```python
from build123d import *

# Parameters (mm, degrees)
EXTRUDE_THIN1_OUTLINE_W   = 1485.9
EXTRUDE_THIN1_OUTLINE_H   = 1041.4
EXTRUDE_THIN1_OUTLINE_W_2 = 228.6
EXTRUDE_THIN1_OUTLINE_H_2 = 228.6
EXTRUDE_THIN1_OUTLINE_W_3 = 355.6
EXTRUDE_THIN1_OUTLINE_H_3 = 482.6
EXTRUDE_THIN1_DEPTH       = 304.8
SKETCH1_5_W               = 1460.5
SKETCH1_5_H               = 1016
BOSS_EXTRUDE1_DEPTH       = 2.54
CUT_EXTRUDE1_DEPTH        = 25.4
SKETCH4_W                 = 127
SKETCH4_H                 = 228.6
CUT_EXTRUDE2_DEPTH        = 25.4
SKETCH5_W                 = 127
SKETCH5_H                 = 228.6
CUT_EXTRUDE3_DEPTH        = 25.4
SKETCH6_W                 = 127
SKETCH6_H                 = 228.6
CUT_EXTRUDE4_DEPTH        = 25.4


# Read off the part's stored shape, not the designer's step: Extrude-Thin1
with BuildPart() as part:
    # Extrude-Thin1 outline → Extrude-Thin1 (new body)
    with BuildSketch(Plane(origin=(0, 0, 0), x_dir=(1, 0, 0), z_dir=(0, 1, 0))):
        Rectangle(EXTRUDE_THIN1_OUTLINE_W, EXTRUDE_THIN1_OUTLINE_H)
        with Locations((222.25, -381)):
            Rectangle(EXTRUDE_THIN1_OUTLINE_W_2, EXTRUDE_THIN1_OUTLINE_H_2, mode=Mode.SUBTRACT)
        with Locations((539.75, -254)):
            Rectangle(EXTRUDE_THIN1_OUTLINE_W_3, EXTRUDE_THIN1_OUTLINE_H_3, mode=Mode.SUBTRACT)
        Polygon((-44.45, 495.3), (-44.45, 241.3), (336.55, 241.3), (336.55, -241.3), (82.55, -241.3), (82.55, -495.3), (-717.55, -495.3), (-717.55, 495.3), align=None, mode=Mode.SUBTRACT)
        with Locations((539.75, 254)):
            Rectangle(EXTRUDE_THIN1_OUTLINE_W_3, EXTRUDE_THIN1_OUTLINE_H_3, mode=Mode.SUBTRACT)
        with Locations((158.75, 381)):
            Rectangle(EXTRUDE_THIN1_OUTLINE_W_3, EXTRUDE_THIN1_OUTLINE_H_2, mode=Mode.SUBTRACT)
    extrude(amount=EXTRUDE_THIN1_DEPTH)

    # Sketch1<5> → Boss-Extrude1 (add)
    with BuildSketch(Plane(origin=(0, 0, 0), x_dir=(1, 0, 0), z_dir=(0, 1, 0))):
        Rectangle(SKETCH1_5_W, SKETCH1_5_H)
    extrude(amount=BOSS_EXTRUDE1_DEPTH)

    # Sketch2 → Cut-Extrude1 (cut)
    with BuildSketch(Plane.ZY.offset(742.95)):
        Polygon((-63.5, 0), (-63.5, 228.6), (63.5, 228.6), (63.5, 0), (0, 0), align=None)
    extrude(amount=-CUT_EXTRUDE1_DEPTH, mode=Mode.SUBTRACT)

    # Sketch4 → Cut-Extrude2 (cut)
    with BuildSketch(Plane.ZY.offset(-336.55)):
        with Locations((-127, 116.84)):
            Rectangle(SKETCH4_W, SKETCH4_H)
        with Locations((127, 116.84)):
            Rectangle(SKETCH4_W, SKETCH4_H)
    extrude(amount=-CUT_EXTRUDE2_DEPTH, mode=Mode.SUBTRACT)

    # Sketch5 → Cut-Extrude3 (cut)
    with BuildSketch(Plane(origin=(0, 0, 241.3), x_dir=(-1, 0, 0), z_dir=(0, 0, -1))):
        with Locations((-209.55, 116.84)):
            Rectangle(SKETCH5_W, SKETCH5_H)
    extrude(amount=-CUT_EXTRUDE3_DEPTH, mode=Mode.SUBTRACT)

    # Sketch6 → Cut-Extrude4 (cut)
    with BuildSketch(Plane.XY.offset(-241.3)):
        with Locations((82.55, 116.84)):
            Rectangle(SKETCH6_W, SKETCH6_H)
    extrude(amount=-CUT_EXTRUDE4_DEPTH, mode=Mode.SUBTRACT)


solid = part.part
```
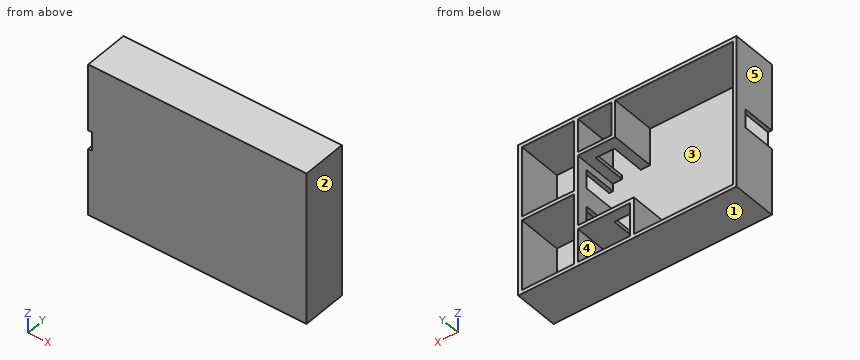
Build history of the part. All positions in model axes, mm. Face numbers are marked on the shaded views. A direction names the side the tool comes from. Round coordinates to 2 decimals unless told otherwise and drop trailing zeros. Order: outer loops, then holes, each group sorted by start corner. A loop starts at its lowest first (then second) coordinate and runs counter-clockwise, first axis right, second up. Notation, with made-up numbers: (85.25, 63.5) - (102.25, 63.5) arc R13 cw to (102.25, 75.5) - close; hole circle Ø7 at (-3.75, 36). An arc over 180 degrees is marked (long way). Use a Markdown table: item, result.
1) Flat gauge pins, fed straight in: pin 1 Ø2 at (x, z) = (545, 288.5) entering from +Y; pin 2 Ø2 at (y, z) = (2, 29.5) entering from -X. Where does each tip first touch, or does it go through?
Recorded:
| item | result |
|---|---|
| pin 1 | stops at y = 2.54 |
| pin 2 | stops at x = -717.55 |
2) Saw through at C-C on y = 248.5. Write the cut outline in (x, z), and give its area (3 significant figures).
Recorded:
| item | result |
|---|---|
| outline | (-742.95, -520.7) - (742.95, -520.7) - (742.95, 520.7) - (-742.95, 520.7) - close; hole (-717.55, -495.3) - (-44.45, -495.3) - (-44.45, -241.3) - (336.55, -241.3) - (336.55, 241.3) - (82.55, 241.3) - (82.55, 495.3) - (-717.55, 495.3) - close; hole (-19.05, -495.3) - (336.55, -495.3) - (336.55, -266.7) - (-19.05, -266.7) - close; hole (107.95, 266.7) - (336.55, 266.7) - (336.55, 495.3) - (107.95, 495.3) - close; hole (361.95, -495.3) - (717.55, -495.3) - (717.55, -12.7) - (361.95, -12.7) - close; hole (361.95, 12.7) - (717.55, 12.7) - (717.55, 495.3) - (361.95, 495.3) - close |
| area | 188,000 mm² |
3) Saw through at A-A on z = 162.5. Write the cut outline in (x, y), and give its area (3 significant figures).
Recorded:
| item | result |
|---|---|
| outline | (-742.95, 0) - (742.95, 0) - (742.95, 304.8) - (717.55, 304.8) - (717.55, 2.54) - (-717.55, 2.54) - (-717.55, 304.8) - (-742.95, 304.8) - close; (336.55, 231.14) - (361.95, 231.14) - (361.95, 304.8) - (336.55, 304.8) - close |
| area | 21,000 mm² |
4) Pull direction X, two halves, no side cores. Call the marked faces 1, 2 and 3: pulls with the +X half, pulls with the -X half, needs draft (parallel to the pull), parting line crosses it, or undercut.
Recorded:
| item | result |
|---|---|
| face 1 | needs draft |
| face 2 | pulls with the +X half |
| face 3 | undercut |
5) Tool access for the marked faces 4 and 5: list every direction of +Z, -Z, +X, -X, +Y, -Y with a clear straight run to the whole face (end or side of a thin tool).
Recorded:
| item | result |
|---|---|
| face 4 | +Y |
| face 5 | +Z, -Z, -X, +Y, -Y |
6) Saw through at B-B on x = 162. Write the cut outline in (y, z).
Recorded:
| item | result |
|---|---|
| outline | (0, -520.7) - (304.8, -520.7) - (304.8, -495.3) - (2.54, -495.3) - (2.54, -266.7) - (304.8, -266.7) - (304.8, -241.3) - (2.54, -241.3) - (2.54, 495.3) - (304.8, 495.3) - (304.8, 520.7) - (0, 520.7) - close; (231.14, 241.3) - (304.8, 241.3) - (304.8, 266.7) - (231.14, 266.7) - close |
7) Wall check: L1, parallel to Z at x = 380, y = 264; L2, parallel to Z at x = 237, y = 20; L3, parallel to X at y = 76, z = 198. Give the ranges that are in metal, low to high.
Recorded:
| item | result |
|---|---|
| L1 | z = -520.7 to -495.3, -12.7 to 12.7, 495.3 to 520.7 |
| L2 | z = -520.7 to -495.3, -266.7 to -241.3, 495.3 to 520.7 |
| L3 | x = -742.95 to -717.55, 336.55 to 361.95, 717.55 to 742.95 |
8) Saw through at D-D on x = 420. Write the cut outline in (y, z), and give its area (3 significant figures).
Recorded:
| item | result |
|---|---|
| outline | (0, -520.7) - (304.8, -520.7) - (304.8, -495.3) - (2.54, -495.3) - (2.54, -12.7) - (304.8, -12.7) - (304.8, 12.7) - (2.54, 12.7) - (2.54, 495.3) - (304.8, 495.3) - (304.8, 520.7) - (0, 520.7) - close |
| area | 25,700 mm² |
